from build123d import *

# Parameters (mm, degrees)
SKETCH1_W                = 82
SKETCH1_H                = 208
BOSS_EXTRUDE1_DEPTH      = 1
F_3_0_3_DIAMETER_HOLE1_D = 3
SKETCH4_W                = 38
SKETCH4_H                = 12
CUT_EXTRUDE1_DEPTH       = 10


with BuildPart() as part:
    # Sketch1 → Boss-Extrude1 (new body)
    with BuildSketch(Plane.XY):
        Rectangle(SKETCH1_W, SKETCH1_H)
    extrude(amount=BOSS_EXTRUDE1_DEPTH)

    # Ø3.0 (3) Diameter Hole1 (through all)
    with Locations(Plane.XY.offset(1)):
        with Locations((-36, 10), (36, 10), (36, -100), (-36, -100), (-36, 100), (36, 100)):
            Hole(F_3_0_3_DIAMETER_HOLE1_D / 2)

    # Sketch4 → Cut-Extrude1 (cut)
    with BuildSketch(Plane.XY.offset(1)):
        with Locations((0, -98)):
            Rectangle(SKETCH4_W, SKETCH4_H)
    extrude(amount=-CUT_EXTRUDE1_DEPTH, mode=Mode.SUBTRACT)


solid = part.part
For this review, take the finished solid that the model builds, in its own axes (mm). Give positions to 0.01 mm unless a question says otherwise; leave off trailing zeros. Order: outer loops, then holes, each group sorted by start corner. A loop starts at its lowest first (then second) coordinate and runs counter-clockwise, first axis right, second up. Notation, with made-up numbers: (-32, -25) - (25, -25) arc R8 cw to (25, -18) - close; hole circle Ø9 at (5, 75). An arc over 180 degrees is marked (long way). Answer as a JSON object with one key per item and string values. Group by question number.
Item 1: Clearance check with flat-ended pins moving along their axes: pin 1 Ø0.5 at (x, z) = (5, 0.5) entering from -Y; pin 2 Ø5 at (x, y) = (36, -100) entering from +Z; pin 3 Ø2.5 at (x, y) = (36, 100) entering from +Z. State where each tip first meets the part, or that it passes through.
Item 2: Take a section at A-A on z = 0.35. Give the boundary of the cut face in (x, y).
Item 3: Wall thickness on line 1 along Y through (x, z) = (36, 0.45); line 2 along X through (y, z) = (100, 0.5); line 3 along X through (y, z) = (-100, 0.3): over which ranges is each line inside the solid? List them lowest first.
Reported:
{
 "1": {"pin 1": "y = -92", "pin 2": "z = 1", "pin 3": "through"},
 "2": {"outline": "(-41, -104) - (-19, -104) - (-19, -92) - (19, -92) - (19, -104) - (41, -104) - (41, 104) - (-41, 104) - close; hole circle Ø3 at (-36, -100); hole circle Ø3 at (-36, 10); hole circle Ø3 at (-36, 100); hole circle Ø3 at (36, -100); hole circle Ø3 at (36, 10); hole circle Ø3 at (36, 100)"},
 "3": {"line 1": "-104 to -101.5, -98.5 to 8.5, 11.5 to 98.5, 101.5 to 104", "line 2": "-41 to -37.5, -34.5 to 34.5, 37.5 to 41", "line 3": "-41 to -37.5, -34.5 to -19, 19 to 34.5, 37.5 to 41"}
}
